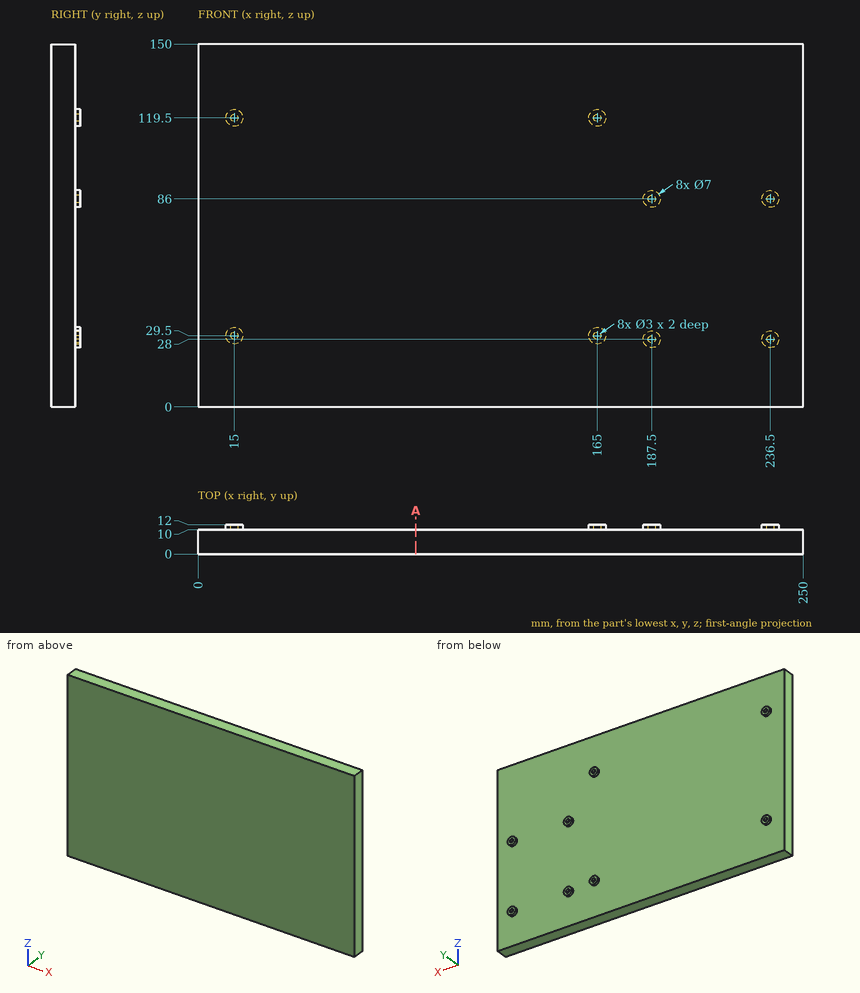
Here's the drawing with two shaded views (mm, measured from the low corner). I have some questions. Give positions to 0.01 mm unless a question says otherwise; leave off trailing zeros. Order: outer loops, then holes, each group sorted by start corner. A loop starts at its lowest first (then second) coordinate and runs counter-clockwise, first axis right, second up.
Q1. I'm going to push a flat-ended pin straight in: P1, Ø1.5, axis at x = 165.5, z = 120, coming from the +Y side. Where does the tip first touch, or does it pass through?
Q2. If I drill on line 1 along Z through (x, y) = (236.5, 10.8); line 2 along Z through (x, y) = (15, 10.85); line 3 along Y through (x, z) = (195, 103), over which ranges is the centre line in solid material (lowest first)?
Q3. Suppose I cut it at A-A, the plane x = 90. Write out the boundary of the cut face in (y, z).
Solution:
1. P1: stops at y = 10
2. line 1: z = 24.5 to 26.5, 29.5 to 31.5, 82.5 to 84.5, 87.5 to 89.5
2. line 2: z = 26 to 28, 31 to 33, 116 to 118, 121 to 123
2. line 3: y = 0 to 10
3. outline: (0, 0) - (10, 0) - (10, 150) - (0, 150) - close
